Design review of the part built by this model. Coordinates are the model's own, in mm. Face numbers are marked on the shaded views. A direction names the side the tool comes from. Round coordinates to 2 decimals unless told otherwise and drop trailing zeros. Loops run counter-clockwise (first coordinate to the right, second up) from the corner with the lowest first, then second, coordinate; pieces in that order, holes last. Notation, with made-up numbers: (21, 50.5) - (73, 50.5) arc R22 ccw to (73, 81.5) - close; hole circle Ø10 at (13.5, 42.25). An arc over 180 degrees is marked (long way). Return JSON: item names as keys, results as strings. Group by question number.
(1) We need section B-B, the plane z = -20. Write out the cut boundary in (x, y), and give its area (3 significant figures).
(2) We need section A-A, the plane y = -23.5. Write out the cut boundary in (x, z), and give its area (3 significant figures).
(3) Clearance check with flat-ended pins moving along their axes: pin 1 (1.2 mm diameter, centred on x = -1.5, z = -3, fed in from -Y); pin 2 (2 mm diameter, centred on x = -1.5, y = 1.5, fed in from -Z); pin 3 (1.2 mm diameter, centred on x = -2.5, z = -7, fed in from +Y). State where each tip first meets the part, or that it passes through.
(4) For the marked faces 1, 2 and 3, list the 3-axis set-ups (+Z, -Z, +X, -X, +Y, -Y) from which the entire face can be reached by the end or side of a thin tool; tool diameter is ignored.
(5) We need section D-D, the plane z = -28.5. Write out the cut boundary in (x, y), and give its area (3 significant figures).
(6) The part is to be moulded in two halves that separate along Y. For the marked faces 4, 5, 6 and 7, say which applies: pulls with the +Y half, pulls with the -Y half, needs draft (parallel to the pull), parting line crosses it, or undercut.
(7) Wall thickness on L1, parallel to Y at x = -1.55, z = -32.5; L2, parallel to X at y = -39.25, z = -20; L3, parallel to Y at x = -1.9, z = -12.5: over which ranges is each line inside the solid? List them lowest first. Write a range as [from, to].
(8) We need section C-C, the plane y = -34.5. Write out the cut boundary in (x, z), and give its area (3 significant figures).
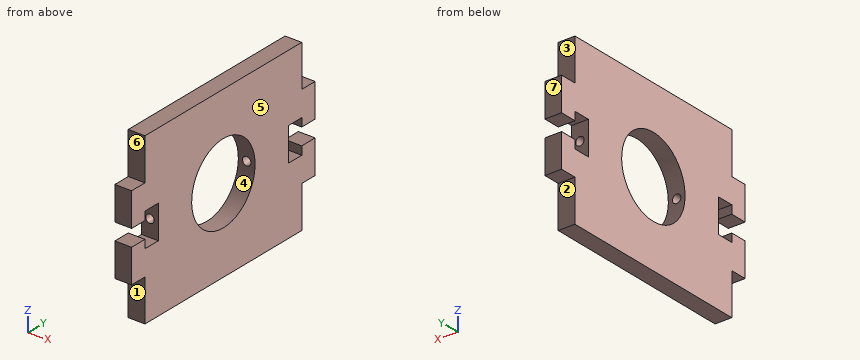
from build123d import *

# Parameters (mm, degrees)
SKETCH_1_R             = 9.5
SM_BASE_FLANGE_1_DEPTH = 4
SKETCH_6_R             = 1
CUT_EXTRUDE_1_DEPTH    = 69.124885321


# Sheet-metal steps are written as plain solids
with BuildPart() as part:
    # Sketch 1 → Базовая кромка1 (new body)
    with BuildSketch(Plane(origin=(0, 0, 0), x_dir=(0, 0, -1), z_dir=(1, 0, 0))):
        Polygon((30, -47), (40, -47), (40, 0), (30, 0), (30, 4), (22, 4), (22, 0), (24, 0), (24, -4), (16, -4), (16, 0), (18, 0), (18, 4), (10, 4), (10, 0), (0, 0), (0, -47), (10, -47), (10, -51), (18, -51), (18, -47), (16, -47), (16, -43), (24, -43), (24, -47), (22, -47), (22, -51), (30, -51), align=None)
        with Locations((20, -23.5)):
            Circle(SKETCH_1_R, mode=Mode.SUBTRACT)
    extrude(amount=-SM_BASE_FLANGE_1_DEPTH)

    # Эскиз6 → Вырез-Вытянуть1 (cut, through all)
    with BuildSketch(Plane(origin=(0, 4, 0), x_dir=(1, 0, 0), z_dir=(0, 1, 0))):
        with Locations(Location((-2, 20, 0), (0, 0, 270))):
            Circle(SKETCH_6_R)
    extrude(amount=-CUT_EXTRUDE_1_DEPTH, mode=Mode.SUBTRACT)


solid = part.part
Solutions:
{
 "1": {"outline": "(-4, -43) - (-3, -43) - (-3, -33) - (-4, -33) - close; (-4, -14) - (-3, -14) - (-3, -4) - (-4, -4) - close; (-1, -43) - (0, -43) - (0, -33) - (-1, -33) - close; (-1, -14) - (0, -14) - (0, -4) - (-1, -4) - close", "area": "40.0 mm^2"},
 "2": {"outline": "(-4, -40) - (0, -40) - (0, -29.5) - (-4, -29.5) - close; (-4, -10.5) - (0, -10.5) - (0, 0) - (-4, 0) - close", "area": "84.0 mm^2"},
 "3": {"pin 1": "y = -47", "pin 2": "z = -30", "pin 3": "y = 0"},
 "4": {"face 1": "-Z, +X, -X, -Y", "face 2": "-Z, +X, -X, +Y", "face 3": "+Z, +X, -X, +Y"},
 "5": {"outline": "(-4, -51) - (0, -51) - (0, -27.74) - (-4, -27.74) - close; (-4, -19.26) - (0, -19.26) - (0, 4) - (-4, 4) - close", "area": "186 mm^2"},
 "6": {"face 4": "undercut", "face 5": "needs draft", "face 6": "pulls with the -Y half", "face 7": "pulls with the +Y half"},
 "7": {"L1": "[-47, 0]", "L2": "[-4, -3], [-1, 0]", "L3": "[-51, -29.33], [-17.67, 4]"},
 "8": {"outline": "(-4, -40) - (0, -40) - (0, 0) - (-4, 0) - close; hole circle Ø2 at (-2, -20)", "area": "157 mm^2"}
}
